Work out the finished part from the listing and answer in its coordinate system (mm). Coordinates: 2 decimals unless noted, no trailing zeros. Write each loop counter-clockwise with the first axis right and the second up, starting at its lowest first coordinate (ties: lowest second). Pieces come first, ordered by that corner, then holes. Notation, with made-up numbers: (80, 6) - (134, 6) arc R14 ccw to (134, 28) - close; hole circle Ø6 at (25.5, -26.5). An arc over 180 degrees is marked (long way). Use CSV: the item, a comma, the result in double quotes. Start each with the question number.
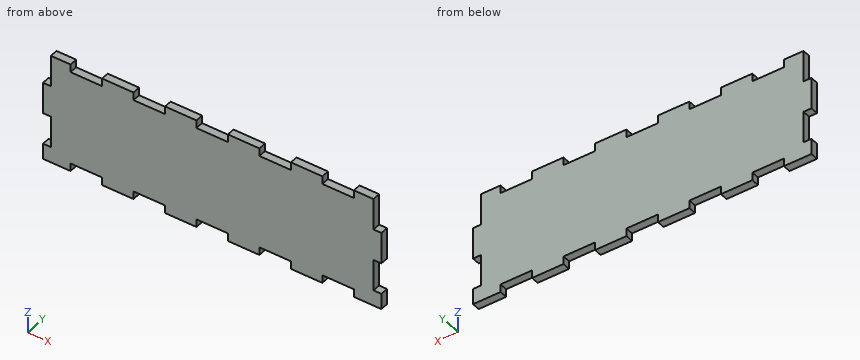
from build123d import *

# Parameters (mm, degrees)
SKETCH_1_W               = 215
SKETCH_1_H               = 70
EXTRUDE_1_DEPTH          = 5
CUT_EXTRUDE_1_REACH      = 115.165
SKETCH_2_W               = 20
SKETCH_2_H               = 5
PATTERN_LINEAR_1_COUNT   = 3
PATTERN_LINEAR_1_PITCH   = 40
PATTERN_LINEAR_2_COUNT   = 3
PATTERN_LINEAR_2_PITCH   = 40
CUT_EXTRUDE_2_REACH      = 115.165
SKETCH_3_W               = 5
SKETCH_3_H               = 20
PATTERN_LINEAR_3_COUNT   = 2
PATTERN_LINEAR_3_PITCH   = 40
MIRROR_1_COPY_1_REACH    = 115.165
MIRROR_1_COPY_1_SKETCH_W = 5
MIRROR_1_COPY_1_SKETCH_H = 20
MIRROR_3_COPY_1_REACH    = 115.165
MIRROR_3_COPY_1_SKETCH_W = 20
MIRROR_3_COPY_1_SKETCH_H = 5
MIRROR_3_COPY_2_REACH    = 115.165
MIRROR_3_COPY_2_SKETCH_W = 20
MIRROR_3_COPY_2_SKETCH_H = 5
MIRROR_3_COPY_3_REACH    = 115.165
MIRROR_3_COPY_3_SKETCH_W = 20
MIRROR_3_COPY_3_SKETCH_H = 5
MIRROR_3_COPY_4_REACH    = 115.165
MIRROR_3_COPY_4_SKETCH_W = 20
MIRROR_3_COPY_4_SKETCH_H = 5


with BuildPart() as part:
    # 스케치1 → 보스-돌출1 (new body)
    with BuildSketch(Plane(origin=(0, 0, 0), x_dir=(1, 0, 0), z_dir=(0, 1, 0))):
        Rectangle(SKETCH_1_W, SKETCH_1_H)
    extrude(amount=EXTRUDE_1_DEPTH)

    # 스케치2 → 컷-돌출1 (cut, up to next)
    with BuildSketch(Plane(origin=(0, 5, 0), x_dir=(1, 0, 0), z_dir=(0, 1, 0)), mode=Mode.PRIVATE) as cut_extrude_1_sk1:
        with Locations((0, -32.5)):
            Rectangle(SKETCH_2_W, SKETCH_2_H)
    cut_extrude_1_tool1 = extrude(cut_extrude_1_sk1.sketch, amount=-CUT_EXTRUDE_1_REACH, mode=Mode.PRIVATE) & part.part
    cut_extrude_1 = cut_extrude_1_tool1.solids().sort_by_distance((0, 5, 32.5))[0]
    add(cut_extrude_1, mode=Mode.SUBTRACT)

    # 선형 패턴1: 컷-돌출1 ×3
    with Locations(*[(i * PATTERN_LINEAR_1_PITCH, 0, 0) for i in range(1, PATTERN_LINEAR_1_COUNT)]):
        add(cut_extrude_1, mode=Mode.SUBTRACT)

    # 선형 패턴2: 컷-돌출1 ×3
    with Locations(*[(-i * PATTERN_LINEAR_2_PITCH, 0, 0) for i in range(1, PATTERN_LINEAR_2_COUNT)]):
        add(cut_extrude_1, mode=Mode.SUBTRACT)

    # 스케치3 → 컷-돌출2 (cut, up to next)
    with BuildSketch(Plane(origin=(0, 5, 0), x_dir=(1, 0, 0), z_dir=(0, 1, 0)), mode=Mode.PRIVATE) as cut_extrude_2_sk1:
        with Locations((105, -25)):
            Rectangle(SKETCH_3_W, SKETCH_3_H)
    cut_extrude_2_tool1 = extrude(cut_extrude_2_sk1.sketch, amount=-CUT_EXTRUDE_2_REACH, mode=Mode.PRIVATE) & part.part
    cut_extrude_2 = cut_extrude_2_tool1.solids().sort_by_distance((105, 5, 25))[0]
    add(cut_extrude_2, mode=Mode.SUBTRACT)

    # 선형 패턴3: 컷-돌출2 ×2
    with Locations(*[(0, 0, -i * PATTERN_LINEAR_3_PITCH) for i in range(1, PATTERN_LINEAR_3_COUNT)]):
        add(cut_extrude_2, mode=Mode.SUBTRACT)

    # 대칭 복사1: 컷-돌출2 across plane
    add(cut_extrude_2.mirror(Plane(origin=(0, 0, 0), x_dir=(0, 0, 1), z_dir=(1, 0, 0))), mode=Mode.SUBTRACT)

    # 대칭 복사1 copy 1 sketch → 대칭 복사1 copy 1 (cut, up to next)
    with BuildSketch(Plane(origin=(0, 5, -40), x_dir=(-1, 0, 0), z_dir=(0, 1, 0)), mode=Mode.PRIVATE) as mirror_1_copy_1_sk1:
        with Locations((105, 25)):
            Rectangle(MIRROR_1_COPY_1_SKETCH_W, MIRROR_1_COPY_1_SKETCH_H)
    mirror_1_copy_1_tool1 = extrude(mirror_1_copy_1_sk1.sketch, amount=-MIRROR_1_COPY_1_REACH, mode=Mode.PRIVATE) & part.part
    add(mirror_1_copy_1_tool1.solids().sort_by_distance((-105, 5, -15))[0], mode=Mode.SUBTRACT)

    # 대칭 복사3: 컷-돌출1 across plane
    add(cut_extrude_1.mirror(Plane.XY), mode=Mode.SUBTRACT)

    # 대칭 복사3 copy 1 sketch → 대칭 복사3 copy 1 (cut, up to next)
    with BuildSketch(Plane(origin=(40, 5, 0), x_dir=(1, 0, 0), z_dir=(0, 1, 0)), mode=Mode.PRIVATE) as mirror_3_copy_1_sk1:
        with Locations((0, 32.5)):
            Rectangle(MIRROR_3_COPY_1_SKETCH_W, MIRROR_3_COPY_1_SKETCH_H)
    mirror_3_copy_1_tool1 = extrude(mirror_3_copy_1_sk1.sketch, amount=-MIRROR_3_COPY_1_REACH, mode=Mode.PRIVATE) & part.part
    add(mirror_3_copy_1_tool1.solids().sort_by_distance((40, 5, -32.5))[0], mode=Mode.SUBTRACT)

    # 대칭 복사3 copy 2 sketch → 대칭 복사3 copy 2 (cut, up to next)
    with BuildSketch(Plane(origin=(80, 5, 0), x_dir=(1, 0, 0), z_dir=(0, 1, 0)), mode=Mode.PRIVATE) as mirror_3_copy_2_sk1:
        with Locations((0, 32.5)):
            Rectangle(MIRROR_3_COPY_2_SKETCH_W, MIRROR_3_COPY_2_SKETCH_H)
    mirror_3_copy_2_tool1 = extrude(mirror_3_copy_2_sk1.sketch, amount=-MIRROR_3_COPY_2_REACH, mode=Mode.PRIVATE) & part.part
    add(mirror_3_copy_2_tool1.solids().sort_by_distance((80, 5, -32.5))[0], mode=Mode.SUBTRACT)

    # 대칭 복사3 copy 3 sketch → 대칭 복사3 copy 3 (cut, up to next)
    with BuildSketch(Plane(origin=(-40, 5, 0), x_dir=(1, 0, 0), z_dir=(0, 1, 0)), mode=Mode.PRIVATE) as mirror_3_copy_3_sk1:
        with Locations((0, 32.5)):
            Rectangle(MIRROR_3_COPY_3_SKETCH_W, MIRROR_3_COPY_3_SKETCH_H)
    mirror_3_copy_3_tool1 = extrude(mirror_3_copy_3_sk1.sketch, amount=-MIRROR_3_COPY_3_REACH, mode=Mode.PRIVATE) & part.part
    add(mirror_3_copy_3_tool1.solids().sort_by_distance((-40, 5, -32.5))[0], mode=Mode.SUBTRACT)

    # 대칭 복사3 copy 4 sketch → 대칭 복사3 copy 4 (cut, up to next)
    with BuildSketch(Plane(origin=(-80, 5, 0), x_dir=(1, 0, 0), z_dir=(0, 1, 0)), mode=Mode.PRIVATE) as mirror_3_copy_4_sk1:
        with Locations((0, 32.5)):
            Rectangle(MIRROR_3_COPY_4_SKETCH_W, MIRROR_3_COPY_4_SKETCH_H)
    mirror_3_copy_4_tool1 = extrude(mirror_3_copy_4_sk1.sketch, amount=-MIRROR_3_COPY_4_REACH, mode=Mode.PRIVATE) & part.part
    add(mirror_3_copy_4_tool1.solids().sort_by_distance((-80, 5, -32.5))[0], mode=Mode.SUBTRACT)


solid = part.part
Item 1: A cutting plane is placed at B-B (x = -74.5). Determine the outline of the cut face in (y, z), then the cut area to 3 significant figures.
Item 2: Straight lines are drawn through the part: probe 1 along X at (y, z) = (1.7, -16); probe 2 along Z at (x, y) = (-79, 1.5). For each, find the intervals that lie inside material, in ascending order. Write a range as [from, to].
Item 3: Each of these flat-tipped pins is pushed along its axis until it touches: pin 1 (1.5 mm diameter, centred on y = 3.5, z = 31.5, fed in from -X); pin 2 (2.5 mm diameter, centred on y = 1.5, z = 32.5, fed in from +X); pin 3 (1.5 mm diameter, centred on x = 41, y = 1.5, fed in from -Z). Where does it stop, or does it pass through?
Item 4: A cutting plane is placed at A-A (z = 21). Determine the outline of the cut face in (x, y), then the cut area to 4 significant figures.
Calculated:
1,outline,"(0, -30) - (5, -30) - (5, 30) - (0, 30) - close"
1,area,"300 mm²"
2,probe 1,"x = [-102.5, 102.5]"
2,probe 2,"z = [-30, 30]"
3,pin 1,"stops at x = -102.5"
3,pin 2,"stops at x = 102.5"
3,pin 3,"stops at z = -30"
4,outline,"(-102.5, 0) - (102.5, 0) - (102.5, 5) - (-102.5, 5) - close"
4,area,"1,025 mm²"
